from build123d import *

# Parameters (mm, degrees)
F0_W     = 8
F0_H     = 130
F1_DEPTH = 4
F2_W     = 4
F2_H     = 126
F3_DEPTH = 2
F4_W     = 4
F4_H     = 35
F5_DEPTH = 2.001


with BuildPart() as f1:
    # F0 (on Top) → F1 (new body)
    with BuildSketch(Plane.XY):
        Rectangle(F0_W, F0_H)
    extrude(amount=F1_DEPTH)

    # F2 (on face) → F3 (cut)
    with BuildSketch(Plane.XY.offset(4)):
        Rectangle(F2_W, F2_H)
    extrude(amount=-F3_DEPTH, mode=Mode.SUBTRACT)

    # F4 (on face) → F5 (cut, through all)
    with BuildSketch(Plane.XY.offset(2)):
        with Locations((0, -29.770957)):
            Rectangle(F4_W, F4_H)
        with Locations((0, 30.229043)):
            Rectangle(F4_W, F4_H)
    extrude(amount=-F5_DEPTH, mode=Mode.SUBTRACT)


solid = f1.part
For this review, take the finished solid that the model builds, in its own axes (mm). A direction names the side the tool comes from. Give positions to 0.01 mm unless a question says otherwise; leave off trailing zeros. Loops run counter-clockwise (first coordinate to the right, second up) from the corner with the lowest first, then second, coordinate; pieces in that order, holes last. Notation, with made-up numbers: (4.25, 54.5) - (61.25, 54.5) arc R3 ccw to (61.25, 59.5) - close; hole circle Ø8 at (57.25, 38). An arc over 180 degrees is marked (long way). Write each question's results on one line, items separated by ' | '.
(1) Draft analysis for pull direction Y (two halves, no side actions). For faces 1 (the flat face through (0, -65, 2)), 2 (the flat face through (0, 1, 0)), 3 (the flat face through (0, 0, 2)), state which applies: +Y half, -Y half, draft (parallel to the pull), parting line (faces both ways), or undercut.
Conclusion:
face 1: -Y half | face 2: draft | face 3: undercut
(2) Take a section at C-C (z = 0.8). Give the boundary of the cut face in (x, y), then the cut area to 3 significant figures.
Conclusion:
outline: (-4, -65) - (4, -65) - (4, 65) - (-4, 65) - close; hole (-2, -47.27) - (2, -47.27) - (2, -12.27) - (-2, -12.27) - close; hole (-2, 12.73) - (2, 12.73) - (2, 47.73) - (-2, 47.73) - close | area: 760 mm^2
(3) Take a section at B-B (y = 46). Give the boundary of the cut face in (x, z), then the cut area to 3 significant figures.
Conclusion:
outline: (-4, 0) - (-2, 0) - (-2, 4) - (-4, 4) - close; (2, 0) - (4, 0) - (4, 4) - (2, 4) - close | area: 16.0 mm^2
(4) For faces 4 (the flat face through (0, 12.729, 1)), 5 (the flat face through (0, -55, 2)), 6 (the flat face through (4, -1, 2)), list the 3-axis set-ups (+Z, -Z, +X, -X, +Y, -Y) from which the entire face can be reached by the end or side of a thin tool; tool diameter is ignored.
Conclusion:
face 4: +Z, -Z | face 5: +Z | face 6: +Z, -Z, +X, +Y, -Y
(5) For line 1 along X through (y, z) = (-35.5, 0.95); line 2 along Y through (x, z) = (-0.75, 0.95); line 3 along Y through (x, z) = (-0.5, 2.35), list the stretches that pass through material, from the lowest coordinate up.
Conclusion:
line 1: -4 to -2, 2 to 4 | line 2: -65 to -47.27, -12.27 to 12.73, 47.73 to 65 | line 3: -65 to -63, 63 to 65
(6) For pin 1 Ø2 at (x, y) = (0.5, -53.5) entering from +Z, flat-tipped, find the tip position at first contact; note if it passes through.
Conclusion:
pin 1: z = 2
(7) Take a section at A-A (x = 0.25). Give the boundary of the cut face in (y, z), then the cut area to 3 significant figures.
Conclusion:
outline: (-65, 0) - (-47.27, 0) - (-47.27, 2) - (-63, 2) - (-63, 4) - (-65, 4) - close; (-12.27, 0) - (12.73, 0) - (12.73, 2) - (-12.27, 2) - close; (47.73, 0) - (65, 0) - (65, 4) - (63, 4) - (63, 2) - (47.73, 2) - close | area: 128 mm^2
